Geometry check sheet. Reference: the model listing, model coordinates, mm. Face numbers are marked on the shaded views. A direction names the side the tool comes from. Give positions to 0.01 mm unless a question says otherwise; leave off trailing zeros. Loops run counter-clockwise (first coordinate to the right, second up) from the corner with the lowest first, then second, coordinate; pieces in that order, holes last. Notation, with made-up numbers: (68, 88.25) -> (81, 88.25) arc R22 cw to (81, 97.25) -> close; hole circle Ø1 at (30, 4). An arc over 180 degrees is marked (long way). Write item = value, one per line.
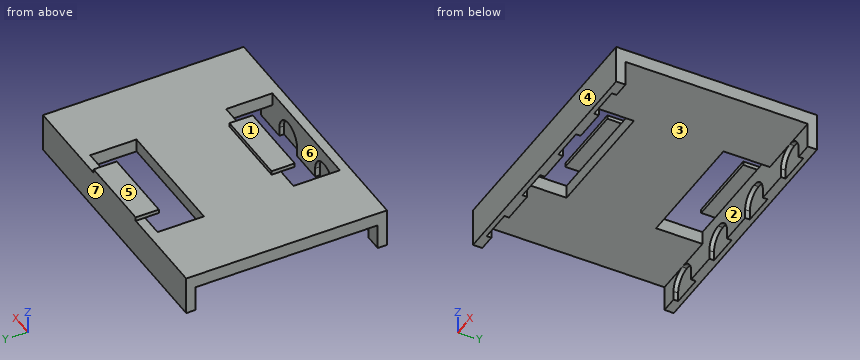
```python
from build123d import *

# Parameters (mm, degrees)
BOSS_EXTRUDE1_DEPTH = 3
BOSS_EXTRUDE2_DEPTH = 3
LPATTERN1_COUNT     = 4
LPATTERN1_PITCH     = 42.5
SKETCH2_W           = 170
SKETCH2_H           = 8.612566395
BOSS_EXTRUDE3_DEPTH = 118
SKETCH4_W           = 2.5
SKETCH4_H           = 15
BOSS_EXTRUDE4_DEPTH = 25
SKETCH4_3_W         = 8.612566395
SKETCH4_3_H         = 30
CUT_EXTRUDE1_DEPTH  = 40


with BuildPart() as part:
    # Sketch1 → Boss-Extrude1 (new body)
    with BuildSketch(Plane(origin=(0, 0, 0), x_dir=(1, 0, 0), z_dir=(0, 1, 0))):
        with BuildLine():
            Line((-21.25, 0), (0, 0))
            Line((0, 0), (0, 8.612566395))
            ThreePointArc((0, 8.612566395), (-7.424621202, 11.687945192), (-10.5, 19.112566395))
            Line((-10.5, 19.112566395), (-10.5, 25.112566395))
            Line((-10.5, 25.112566395), (-21.25, 25.112566395))
            Line((-21.25, 25.112566395), (-21.25, 0))
        make_face()
        with BuildLine():
            Line((0, 8.612566395), (0, 0))
            Line((0, 0), (21.25, 0))
            Line((21.25, 0), (21.25, 25.112566395))
            Line((21.25, 25.112566395), (10.5, 25.112566395))
            Line((10.5, 25.112566395), (10.5, 19.112566395))
            ThreePointArc((10.5, 19.112566395), (7.424621202, 11.687945192), (0, 8.612566395))
        make_face()
        with BuildLine():
            ThreePointArc((-10.5, 19.112566395), (-7.424621202, 11.687945192), (0, 8.612566395))
            Line((0, 8.612566395), (0, 25.112566395))
            Line((0, 25.112566395), (-10.5, 25.112566395))
            Line((-10.5, 25.112566395), (-10.5, 19.112566395))
        make_face()
        with BuildLine():
            Line((0, 25.112566395), (0, 8.612566395))
            ThreePointArc((0, 8.612566395), (7.424621202, 11.687945192), (10.5, 19.112566395))
            Line((10.5, 19.112566395), (10.5, 25.112566395))
            Line((10.5, 25.112566395), (0, 25.112566395))
        make_face()
    boss_extrude1 = extrude(amount=BOSS_EXTRUDE1_DEPTH)

    # Sketch1<3> → Boss-Extrude2 (add)
    with BuildSketch(Plane(origin=(0, 0, 0), x_dir=(1, 0, 0), z_dir=(0, 1, 0))):
        with BuildLine():
            Line((-21.25, 0), (0, 0))
            Line((0, 0), (0, 8.612566395))
            ThreePointArc((0, 8.612566395), (-7.424621202, 11.687945192), (-10.5, 19.112566395))
            Line((-10.5, 19.112566395), (-10.5, 25.112566395))
            Line((-10.5, 25.112566395), (-21.25, 25.112566395))
            Line((-21.25, 25.112566395), (-21.25, 0))
        make_face()
        with BuildLine():
            Line((0, 8.612566395), (0, 0))
            Line((0, 0), (21.25, 0))
            Line((21.25, 0), (21.25, 25.112566395))
            Line((21.25, 25.112566395), (10.5, 25.112566395))
            Line((10.5, 25.112566395), (10.5, 19.112566395))
            ThreePointArc((10.5, 19.112566395), (7.424621202, 11.687945192), (0, 8.612566395))
        make_face()
    boss_extrude2 = extrude(amount=-BOSS_EXTRUDE2_DEPTH)

    # LPattern1: Boss-Extrude1, Boss-Extrude2 ×4
    with Locations(*[(i * LPATTERN1_PITCH, 0, 0) for i in range(1, LPATTERN1_COUNT)]):
        add(boss_extrude1)
        add(boss_extrude2)

    # Sketch2 → Boss-Extrude3 (add)
    with BuildSketch(Plane(origin=(0, -3, 0), x_dir=(-1, 0, 0), z_dir=(0, -1, 0))):
        with Locations((-63.75, 4.306283197)):
            Rectangle(SKETCH2_W, SKETCH2_H)
    extrude(amount=BOSS_EXTRUDE3_DEPTH)

    # Mirror2: part across plane


with BuildPart() as part_1:
    add(part.part)
    add(part.part.mirror(Plane(origin=(0, -62, 0), x_dir=(0, 0, 1), z_dir=(0, -1, 0))))

    # Sketch4 → Boss-Extrude4 (add, symmetric)
    with BuildSketch(Plane.ZY.offset(-63.75)):
        with Locations((1.25, -4.5)):
            Rectangle(SKETCH4_W, SKETCH4_H)
        Polygon((0, -91), (0, -100), (2.5, -100), (2.5, -85), (0, -85), align=None)
    extrude(amount=BOSS_EXTRUDE4_DEPTH, both=True)

    # Sketch4<3> → Cut-Extrude1 (cut, symmetric)
    with BuildSketch(Plane.ZY.offset(-63.75)):
        Polygon((0, -12), (0, -3), (-8.612566395, -3), (-8.612566395, -33), (0, -33), align=None)
        with Locations((-4.306283197, -106)):
            Rectangle(SKETCH4_3_W, SKETCH4_3_H)
    extrude(amount=CUT_EXTRUDE1_DEPTH, both=True, mode=Mode.SUBTRACT)


solid = part_1.part
```
Item 1: Section check C-C, the plane y = -28. Record the cut outline in (x, z).
Answer:
outline = (-21.25, -8.61) -> (23.75, -8.61) -> (23.75, 0) -> (-21.25, 0) -> close; (103.75, -8.61) -> (148.75, -8.61) -> (148.75, 0) -> (103.75, 0) -> close
Item 2: Gauge pin test, flat end, axial feed: pin 1 (12 mm diameter, centred on y = -93, z = -9.5, fed in from +X). Record the tip position at first contact, or that the pin passes through.
Answer:
pin_1 = 148.75
Item 3: Section check A-A, the plane x = 26.5. Record the cut outline in (y, z).
Answer:
outline = (-127, -25.11) -> (-121, -25.11) -> (-121, 0) -> (-127, 0) -> close; (-91, -8.61) -> (-33, -8.61) -> (-33, 0) -> (-91, 0) -> close; (-3, -25.11) -> (3, -25.11) -> (3, 0) -> (-3, 0) -> close
Item 4: Draft check along Y on the marked faces 4, 5, 6 and 7. Enter one of: +Y half, -Y half, draft (parallel to the pull), parting line (faces both ways), or undercut.
Answer:
face_4 = -Y half
face_5 = draft
face_6 = undercut
face_7 = +Y half
Item 5: Section check D-D, the plane z = -5.75. Record the cut outline in (x, y), plus the area to 3 significant figures.
Answer:
outline = (-21.25, -127) -> (148.75, -127) -> (148.75, 3) -> (-21.25, 3) -> close; hole (23.75, -121) -> (103.75, -121) -> (103.75, -91) -> (23.75, -91) -> close; hole (23.75, -33) -> (103.75, -33) -> (103.75, -3) -> (23.75, -3) -> close
area = 17,300 mm^2
Item 6: Tool access check on the marked faces 1, 2 and 3. Record the directions out of +Z, -Z, +X, -X, +Y, -Y that give a thin tool (end or side, any length) a straight path to the whole face; none if there is none.
Answer:
face_1 = +Z, +X, -X, +Y, -Y
face_2 = -Z
face_3 = -Z, +X, -X
Item 7: Thickness scan on L1, parallel to Y at x = 71.5, z = -4.5; L2, parallel to Y at x = 61, z = -19.5; L3, parallel to Y at x = 76, z = -23.5. Record the ranges inside material, lowest first. Write a range as [from, to].
Answer:
L1 = [-127, -121], [-91, -33], [-3, 3]
L2 = [-127, -121], [-3, 3]
L3 = [-127, -124], [0, 3]
Item 8: Section check B-B, the plane y = -93. Record the cut outline in (x, z).
Answer:
outline = (-21.25, -8.61) -> (23.75, -8.61) -> (23.75, 0) -> (-21.25, 0) -> close; (38.75, 0) -> (88.75, 0) -> (88.75, 2.5) -> (38.75, 2.5) -> close; (103.75, -8.61) -> (148.75, -8.61) -> (148.75, 0) -> (103.75, 0) -> close
